Source: three-view drawing plus pictorial views. Frame: mm from the lowest corner of the part. A direction names the side the tool comes from. Coordinates: 2 decimals unless noted, no trailing zeros. Order: outer loops, then holes, each group sorted by start corner. A loop starts at its lowest first (then second) coordinate and runs counter-clockwise, first axis right, second up. Notation, with made-up numbers: (70, -12.75) -> (97, -12.75) arc R18 cw to (97, -6.75) -> close; hole circle Ø6 at (-9.75, 22.25). An arc over 180 degrees is marked (long way). Use one line per item in the form item = value. Start each with the question number.
1) Ray query, line 1 along Y through (x, z) = (6, 5); line 2 along Z through (x, y) = (5.5, 7.5); line 3 along Z through (x, y) = (6, 8). Return the intervals inside material, ascending.
2) Section query B-B on z = 5. Output: boundary loops of the cut face in (x, y), then the cut area to 3 significant figures.
3) Section query C-C on x = 1.25. Output: boundary loops of the cut face in (y, z), then the cut area to 3 significant figures.
4) Pin query (flat end, axial travel): pin 1 (1.6 mm diameter, centred on x = 1, y = 8.5, fed in from +Z); pin 2 (3 mm diameter, centred on y = 8, z = 13, fed in from -X). Return the tip coordinate at first contact, or that it passes through.
5) Section query A-A on y = 7.5. Output: boundary loops of the cut face in (x, z).
6) Section query D-D on y = 2.5. Output: boundary loops of the cut face in (x, z).
7) Access query for the marked faces 1 and 2. Directions: +Z, -Z, +X, -X, +Y, -Y. A direction counts if a zero-diameter tool reaches every point of the face in a straight line with its end or side. Return the directions, or none.
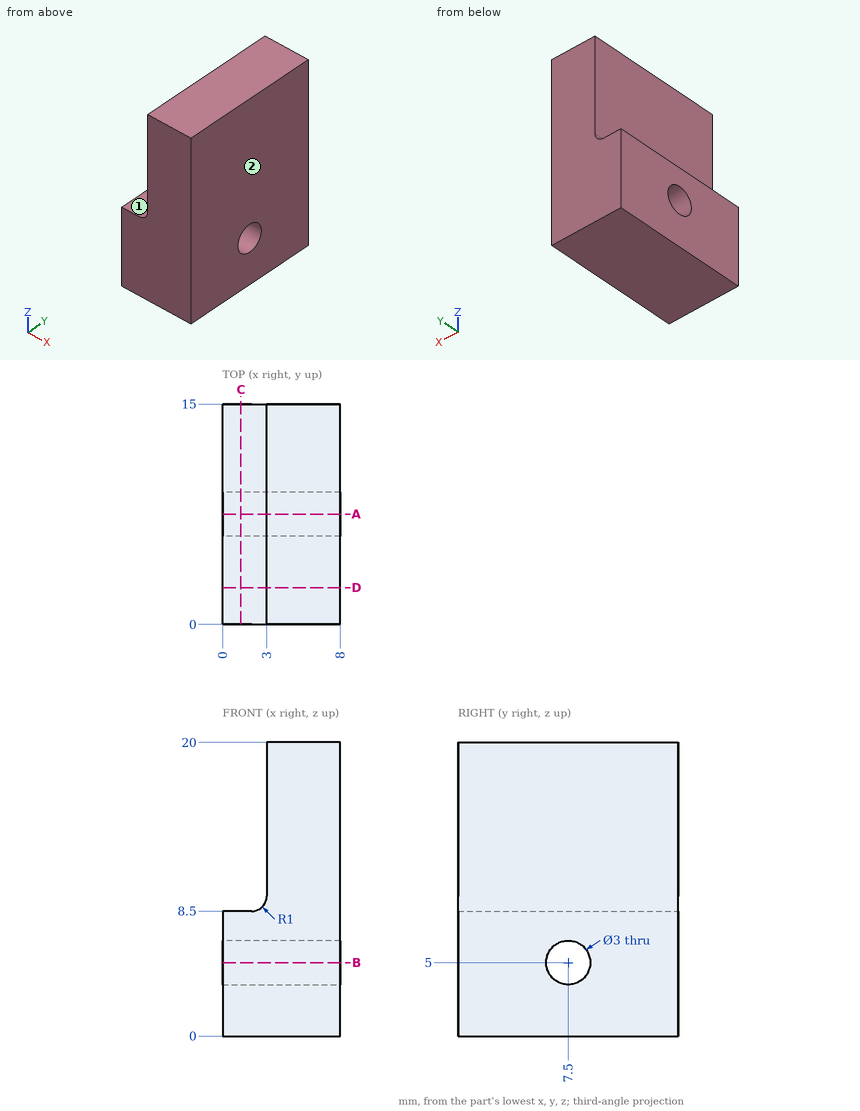
Answers below:
q1.line_1 = 0 to 6, 9 to 15
q1.line_2 = 0 to 3.5, 6.5 to 20
q1.line_3 = 0 to 3.59, 6.41 to 20
q2.outline = (0, 0) -> (8, 0) -> (8, 6) -> (0, 6) -> close; (0, 9) -> (8, 9) -> (8, 15) -> (0, 15) -> close
q2.area = 96.0 mm^2
q3.outline = (0, 0) -> (15, 0) -> (15, 8.5) -> (0, 8.5) -> close; hole circle Ø3 at (7.5, 5)
q3.area = 120 mm^2
q4.pin_1 = 8.5
q4.pin_2 = 3
q5.outline = (0, 0) -> (8, 0) -> (8, 3.5) -> (0, 3.5) -> close; (0, 6.5) -> (8, 6.5) -> (8, 20) -> (3, 20) -> (3, 9.5) arc R1 cw to (2, 8.5) -> (0, 8.5) -> close
q6.outline = (0, 0) -> (8, 0) -> (8, 20) -> (3, 20) -> (3, 9.5) arc R1 cw to (2, 8.5) -> (0, 8.5) -> close
q7.face_1 = +Z, -X, +Y, -Y
q7.face_2 = +Z, -Z, +X, +Y, -Y
